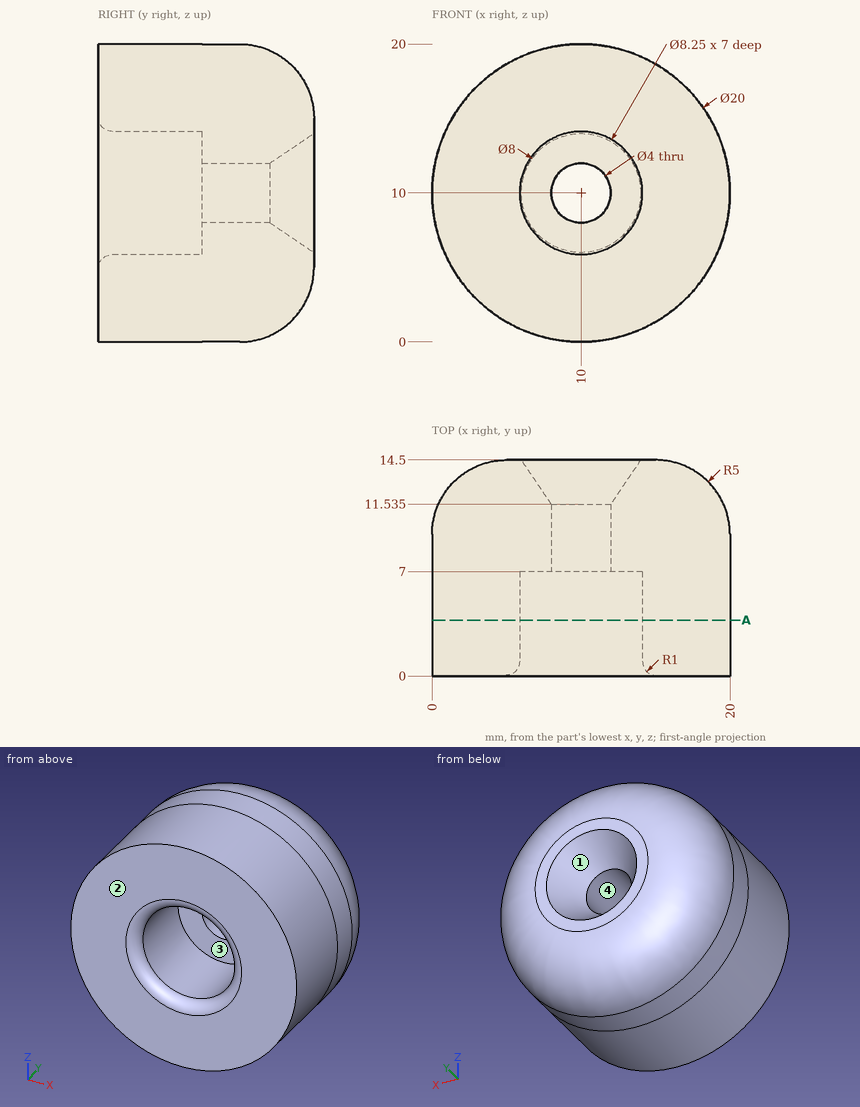
Check sheet for the drawn part. Datum: minimum x, y, z corner. Units: mm. A direction names the side the tool comes from. Coordinates: 2 decimals unless noted, no trailing zeros. Order: outer loops, then holes, each group sorted by start corner. A loop starts at its lowest first (then second) coordinate and runs counter-clockwise, first axis right, second up. Notation, with made-up numbers: (49, 13.25) -> (76, 13.25) arc R24 cw to (76, 31.25) -> close; hole circle Ø6 at (59, -16). An arc over 180 degrees is marked (long way). Use a Markdown table: item, result. Add a question column.
1. Cross-section at A-A (y = 3.75). Enter the section's corners in (x, z) (3 decimals), and give its area (3 significant figures).
2. Set-up check for the marked faces 3 and 4: record each of +Z, -Z, +X, -X, +Y, -Y from which the full face is reachable in a straight line by a thin tool's end or side.
3. Go/stop test with flat-tipped pins: pin 1 Ø4 at (x, y) = (13, 7) entering from -Z; pin 2 Ø1 at (x, y) = (3, 7.5) entering from +Z; pin 3 Ø5 at (x, z) = (3.5, 15) entering from +Y; pin 4 Ø2.5 at (x, z) = (10, 10) entering from -Y. Record where each tip stops, or that it passes through.
4. Material ranges on L1, parallel to X at y = 9.4, z = 10; L2, parallel to X at y = 5.2, z = 10 (3 decimals), recorded low to high.
5. Mould release check, pull along X, two halves, no side actions. Record for the marked faces 1 and 2: pulls with the +X half, pulls with the -X half, needs draft (parallel to the pull), parting line crosses it, or undercut.
Filled sheet:
| question | item | result |
|---|---|---|
| 1 | outline | circle Ø20 at (10, 10); hole circle Ø8.25 at (10, 10) |
| 1 | area | 261 mm2 |
| 2 | face 3 | -Y |
| 2 | face 4 | +Y, -Y |
| 3 | pin 1 | z = 0.05 |
| 3 | pin 2 | z = 17.6 |
| 3 | pin 3 | y = 14.45 |
| 3 | pin 4 | through |
| 4 | L1 | 0 to 8, 12 to 20 |
| 4 | L2 | 0 to 5.875, 14.125 to 20 |
| 5 | face 1 | undercut |
| 5 | face 2 | needs draft |
